```python
from build123d import *

# Parameters (mm, degrees)
SKETCH_1_W          = 70
SKETCH_1_H          = 50
EXTRUDE_1_DEPTH     = 2
SKETCH_2_W          = 11.266192233
SKETCH_2_H          = 8.432364739
SKETCH_2_W_2        = 11.75001644
SKETCH_2_H_2        = 6.220596939
EXTRUDE_2_DEPTH     = 8
SKETCH_3_R          = 2.073259277
SKETCH_3_W          = 5.968463231
SKETCH_3_H          = 1.961690003
SKETCH_3_H_2        = 1.772031982
CUT_EXTRUDE_1_DEPTH = 8


with BuildPart() as part:
    # 草图1 → 凸台-拉伸1 (new body)
    with BuildSketch(Plane(origin=(0, 0, 0), x_dir=(1, 0, 0), z_dir=(0, 1, 0))):
        with Locations((12.700831025, -15.40166205)):
            Rectangle(SKETCH_1_W, SKETCH_1_H)
    extrude(amount=EXTRUDE_1_DEPTH)

    # 草图2 → 凸台-拉伸2 (add)
    with BuildSketch(Plane(origin=(0, 2, 0), x_dir=(1, 0, 0), z_dir=(0, 1, 0))):
        with Locations((-20.302891623, -0.16119955)):
            Rectangle(SKETCH_2_W, SKETCH_2_H)
        with Locations((-20.060979519, -30.503889063)):
            Rectangle(SKETCH_2_W_2, SKETCH_2_H_2)
    extrude(amount=EXTRUDE_2_DEPTH)

    # 草图3 → 切除-拉伸1 (cut)
    with BuildSketch(Plane.ZY.offset(25.935987739)):
        with Locations((30.500300108, 5.554053281)):
            Circle(SKETCH_3_R)
        with Locations((0.41832149, 4.57320828)):
            Rectangle(SKETCH_3_W, SKETCH_3_H)
        with Locations((0.41832149, 7.612359017)):
            Rectangle(SKETCH_3_W, SKETCH_3_H_2)
    extrude(amount=-CUT_EXTRUDE_1_DEPTH, mode=Mode.SUBTRACT)


solid = part.part
```
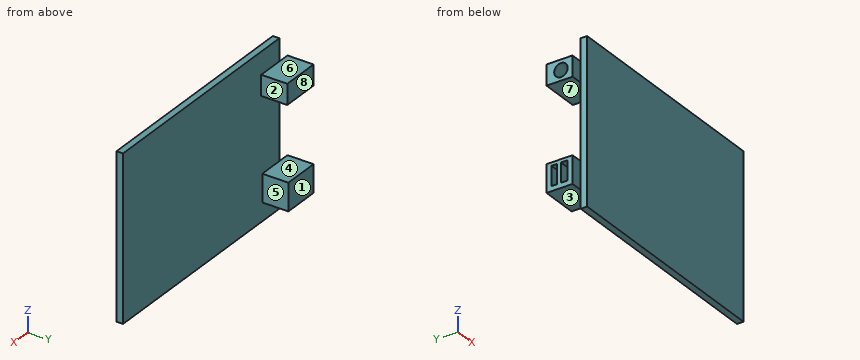
Can you work these out from the model? Positions are in its coordinate system, mm. Face numbers are marked on the shaded views. A direction names the side the tool comes from. Give positions to 0.01 mm unless a question says otherwise; leave off trailing zeros. Loops run counter-clockwise (first coordinate to the right, second up) from the corner with the lowest first, then second, coordinate; pieces in that order, holes last. Notation, with made-up numbers: M 11,-33.5 L 26,-33.5 A29 ccw 26,5.5 Z; hole C 38,79 d7. An arc over 180 degrees is marked long. One line per question, with ' | ' between items. Start each with the question number.
Q1. If we section it at A-A (y = 4.75): Please give me the cut outline in (x, z), plus the area to 3 significant figures.
Q2. If we section it at B-B (z = 1.5): Please give me the cut outline in (x, y).
Q3. For pin 1 Ø1.4 at (y, z) = (7.5, 1.5) entering from -X; pin 2 Ø6 at (x, z) = (-8.5, -3.5) entering from +Y; pin 3 Ø1.4 at (x, y) = (-21, 7.5) entering from -Z (3 decimals), each with a flat end and sliding along its axis, tell me the tip position at first contact or that it passes through.
Q4. For the marked faces 1, 2, 3, 4 and 5, which set-ups out of +Z, -Z, +X, -X, +Y, -Y let a thin tool reach every point of the face, with its end or its side?
Q5. If we section it at C-C (x = -17): Please give me the cut outline in (y, z).
Q6. If we section it at D-D (z = 9): Please give me the cut outline in (x, y), plus the area to 3 significant figures.
Q7. If I drill on line 1 (Y direction, x = 10, z = 13); line 2 (X direction, y = 1.5, z = 1); line 3 (Z direction, x = -16, y = 6), over which ranges is the centre line in solid material (lowest first)? Write a range as from..to.
Q8. If we mould it in two halves opening along Z, with no side actions, what happens to the marked faces 6, 7 and 8? For each: +Z half, -Z half, draft (parallel to the pull), parting line (faces both ways), or undercut.
Computed:
1) outline: M -25.94,-4.05 L -14.67,-4.05 L -14.67,4.38 L -25.94,4.38 L -25.94,3.4 L -17.94,3.4 L -17.94,-2.57 L -25.94,-2.57 Z; M -25.94,27.39 L -14.19,27.39 L -14.19,33.61 L -25.94,33.61 L -25.94,32.41 L -17.94,32.41 L -17.94,28.59 L -25.94,28.59 Z | area: 89.8 mm²
2) outline: M -25.94,2 L -22.3,2 L -22.3,0 L 47.7,0 L 47.7,2 L -14.67,2 L -14.67,10 L -25.94,10 L -25.94,8.5 L -17.94,8.5 L -17.94,6.73 L -25.94,6.73 L -25.94,5.55 L -17.94,5.55 L -17.94,3.59 L -25.94,3.59 Z
3) pin 1: stops at x = -17.94 | pin 2: stops at y = 2 | pin 3: stops at z = -4.055
4) face 1: +Z, -Z, +X, -X, +Y | face 2: +Z, -Z, +X, +Y | face 3: -Z, +X, -X, +Y | face 4: +X, -X, +Y | face 5: -Z, +X, +Y
5) outline: M 0,-9.6 L 2,-9.6 L 2,-4.05 L 10,-4.05 L 10,4.38 L 2,4.38 L 2,27.39 L 10,27.39 L 10,33.61 L 2,33.61 L 2,40.4 L 0,40.4 Z
6) outline: M -22.3,0 L 47.7,0 L 47.7,2 L -22.3,2 Z | area: 140 mm²
7) line 1: y = 0..2 | line 2: x = -22.3..47.7 | line 3: z = -4.05..4.38, 27.39..33.61
8) face 6: +Z half | face 7: undercut | face 8: draft
